```python
from build123d import *

# Parameters (mm, degrees)
BOSS_EXTRUDE2_DEPTH = 10
SKETCH3_R           = 50
BOSS_EXTRUDE3_DEPTH = 10
SKETCH4_R           = 10
BOSS_EXTRUDE4_DEPTH = 90
CUT_EXTRUDE1_START  = -30
SKETCH5_R           = 10
CUT_EXTRUDE1_DEPTH  = 30
SKETCH6_R           = 13
CUT_EXTRUDE2_DEPTH  = 10
SKETCH7_R           = 10
BOSS_EXTRUDE5_DEPTH = 30
SKETCH8_R           = 20.369169003
BOSS_EXTRUDE6_DEPTH = 10
CUT_EXTRUDE3_START  = -100
SKETCH9_R           = 10
CUT_EXTRUDE3_DEPTH  = 100
SKETCH10_R          = 10
CUT_EXTRUDE4_DEPTH  = 10
SKETCH11_R          = 12.5
CUT_EXTRUDE5_DEPTH  = 10
SCALE1_SCALE        = 0.2


with BuildPart() as part:
    # Sketch1 → Boss-Extrude2 (new body)
    with BuildSketch(Plane.XY):
        Polygon((20, 144), (-20, 144), (-20, 11.547005384), (-134.707658145, -54.679491924), (-114.707658145, -89.320508076), (0, -23.094010768), (114.707658145, -89.320508076), (134.707658145, -54.679491924), (20, 11.547005384), align=None)
    extrude(amount=BOSS_EXTRUDE2_DEPTH)

    # Sketch3 → Boss-Extrude3 (add)
    with BuildSketch(Plane.XY.offset(10)):
        with Locations((-124.707658145, -72)):
            Circle(SKETCH3_R)
        with Locations((0, 144)):
            Circle(SKETCH3_R)
        with Locations((124.707658145, -72)):
            Circle(SKETCH3_R)
    extrude(amount=-BOSS_EXTRUDE3_DEPTH)

    # Sketch4 → Boss-Extrude4 (add)
    with BuildSketch(Plane.XY.offset(10)):
        with Locations(Location((0, 144, 0), (0, 0, 180))):
            Circle(SKETCH4_R)
        with Locations(Location((124.707658145, -72, 0), (0, 0, 180))):
            Circle(SKETCH4_R)
        with Locations(Location((-124.707658145, -72, 0), (0, 0, 180))):
            Circle(SKETCH4_R)
    extrude(amount=BOSS_EXTRUDE4_DEPTH)

    # Sketch5 → Cut-Extrude1 (cut)
    with BuildSketch(Plane.XY.offset(100).offset(CUT_EXTRUDE1_START)):
        with Locations(Location((0, 144, 0), (0, 0, 180))):
            Circle(SKETCH5_R)
    extrude(amount=CUT_EXTRUDE1_DEPTH, mode=Mode.SUBTRACT)

    # Sketch6 → Cut-Extrude2 (cut)
    with BuildSketch(Plane.XY.offset(10)):
        Circle(SKETCH6_R)
    extrude(amount=-CUT_EXTRUDE2_DEPTH, mode=Mode.SUBTRACT)

    # Sketch7 → Boss-Extrude5 (add)
    with BuildSketch(Plane.XY.offset(70)):
        with Locations(Location((0, 144, 0), (0, 0, 180))):
            Circle(SKETCH7_R)
    extrude(amount=BOSS_EXTRUDE5_DEPTH)

    # Sketch8 → Boss-Extrude6 (add)
    with BuildSketch(Plane.XY.offset(10)):
        Circle(SKETCH8_R)
    extrude(amount=-BOSS_EXTRUDE6_DEPTH)

    # Sketch9 → Cut-Extrude3 (cut)
    with BuildSketch(Plane.XY.offset(100).offset(CUT_EXTRUDE3_START)):
        with Locations((-124.707658145, -72)):
            Circle(SKETCH9_R)
        with Locations((0, 144)):
            Circle(SKETCH9_R)
        with Locations((124.707658145, -72)):
            Circle(SKETCH9_R)
    extrude(amount=CUT_EXTRUDE3_DEPTH, mode=Mode.SUBTRACT)

    # Sketch10 → Cut-Extrude4 (cut)
    with BuildSketch(Plane.XY.offset(10)):
        Circle(SKETCH10_R)
    extrude(amount=-CUT_EXTRUDE4_DEPTH, mode=Mode.SUBTRACT)

    # Sketch11 → Cut-Extrude5 (cut)
    with BuildSketch(Plane.XY.offset(10)):
        Circle(SKETCH11_R)
    extrude(amount=-CUT_EXTRUDE5_DEPTH, mode=Mode.SUBTRACT)


with BuildPart() as part_1:
    # Scale1: scaled about (0, 0, 5)
    add(part.part.scale(SCALE1_SCALE).moved(Location((0, 0, 4))))


solid = part_1.part
```
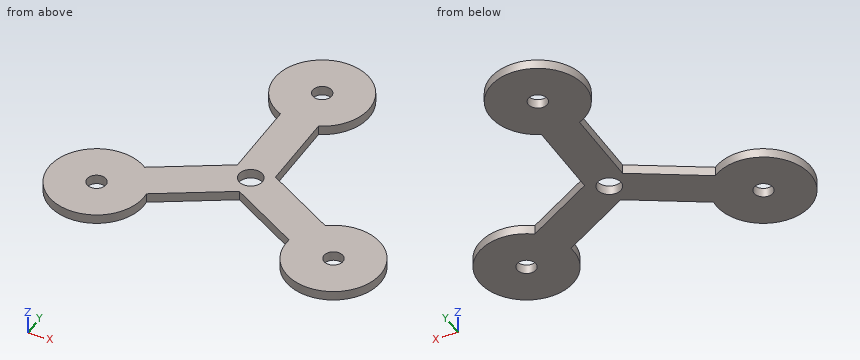
Verification items for the finished model (mm, model axes). Coordinates: 2 decimals unless noted, no trailing zeros. Loops run counter-clockwise (first coordinate to the right, second up) from the corner with the lowest first, then second, coordinate; pieces in that order, holes last. Notation, with made-up numbers: (50, -34) -> (74, -34) arc R21 ccw to (74, -13) -> close; hole circle Ø4 at (-30.75, -16). An arc over 180 degrees is marked (long way). Answer in a Markdown table with one row per item. Add a question column.
1. Section check B-B, the plane z = 5.1. Enter the section's corners in (x, y).
2. Section check C-C, the plane x = -8.5. Enter the section's corners in (y, z).
3. Material ranges on probe 1 along X at (y, z) = (-14.4, 4.8); probe 2 along Y at (x, z) = (0, 4.4); probe 3 along Y at (x, z) = (-25, 4.5), recorded low to high. Write a range as [from, to].
4. Section check D-D, the plane y = 15. Enter the section's corners in (x, z), then the cut area to 3 significant figures.
5. Section check A-A, the plane y = 0. Enter the section's corners in (x, z).
6. Depth check by flat-ended pin: P1, Ø1, axis at y = 19.5, z = 4.5, coming from the +X side; P2, Ø0.6, axis at y = 8.5, z = 4.5, coming from the +X side; P3, Ø2.5, axis at x = 24.94, y = -14.4, coming from the +Z side. Enter the tip coordinate at first touch or a pass-through.
Derived:
| question | item | result |
|---|---|---|
| 1 | outline | (-19, -6.35) arc R10 ccw (long way) to (-15, -13.28) -> (0, -4.62) -> (15, -13.28) arc R10 ccw (long way) to (19, -6.35) -> (4, 2.31) -> (4, 19.63) arc R10 ccw (long way) to (-4, 19.63) -> (-4, 2.31) -> close; hole circle Ø4 at (-24.94, -14.4); hole circle Ø5 at (0, 0); hole circle Ø4 at (0, 28.8); hole circle Ø4 at (24.94, -14.4) |
| 2 | outline | (-9.53, 4) -> (-0.29, 4) -> (-0.29, 6) -> (-9.53, 6) -> close; (23.53, 4) -> (34.07, 4) -> (34.07, 6) -> (23.53, 6) -> close |
| 3 | probe 1 | x = [-34.94, -26.94], [-22.94, -14.94], [14.94, 22.94], [26.94, 34.94] |
| 3 | probe 2 | y = [-4.62, -2.5], [2.5, 26.8], [30.8, 38.8] |
| 3 | probe 3 | y = [-24.4, -16.4], [-12.4, -4.4] |
| 4 | outline | (-4, 4) -> (4, 4) -> (4, 6) -> (-4, 6) -> close |
| 4 | area | 16.0 mm² |
| 5 | outline | (-8, 4) -> (-2.5, 4) -> (-2.5, 6) -> (-8, 6) -> close; (2.5, 4) -> (8, 4) -> (8, 6) -> (2.5, 6) -> close |
| 6 | P1 | stops at x = 4.75 |
| 6 | P2 | stops at x = 4 |
| 6 | P3 | passes through |
